Geometry check sheet. Reference: the model listing, model coordinates, mm. A direction names the side the tool comes from. Round coordinates to 2 decimals unless told otherwise and drop trailing zeros. Order: outer loops, then holes, each group sorted by start corner. A loop starts at its lowest first (then second) coordinate and runs counter-clockwise, first axis right, second up. Notation, with made-up numbers: (84.25, 87) - (100.25, 87) arc R25 cw to (100.25, 112) - close; hole circle Ø11 at (74.5, -31.75). An arc over 180 degrees is marked (long way). Return JSON: item names as keys, results as strings. Group by question number.
Q1. Sectioned sample at A-A, the plane y = -41. Record the cut outline in (x, z) (3 decimals).
Q2. Material ranges on line 1 along Y through (x, z) = (41, 2.75) (3 decimals); line 2 along Y through (x, z) = (-21, 9); line 3 along Y through (x, z) = (-23.5, 3), recorded low to high.
Q3. Gauge pin test, flat ends, axial feed: pin 1 Ø2 at (x, z) = (53, 1.5) entering from -Y; pin 2 Ø4 at (x, z) = (20.5, 5) entering from +Y; pin 3 Ø1 at (y, z) = (19, 5.5) entering from -X. Record the tip position at first contact, or that the pin passes through.
Q4. Sectioned sample at C-C, the plane x = -41. Record the cut outline in (y, z) (3 decimals), then the cut area to 3 significant figures.
Q5. Draft check along X on faces 1 (the flat face through (-45, 1, 5)), 2 (the flat face through (1, 45, 6)), 3 (the flat face through (-21.75, -20, 5)). Enter one of: pulls with the +X half, pulls with the -X half, needs draft (parallel to the pull), parting line crosses it, or undercut.
Q6. Tool access check on faces 4 (the flat face through (20, -18.25, 5)), 5 (the flat face through (45, -1, 5)), 6 (the flat face through (-1, 30, 0)). Record the directions out of +Z, -Z, +X, -X, +Y, -Y that give a thin tool (end or side, any length) a straight path to the whole face; none if there is none.
Q7. Sectioned sample at B-B, the plane z = 5. Give the number of separate pieces and of enclosed holes in the cut face, then the cut area to 3 significant figures.
Q8. Sectioned sample at D-D, the plane x = 12.5. Record the cut outline in (y, z), then the cut area to 4 significant figures.
```python
from build123d import *

# Parameters (mm, degrees)
F0_R     = 1.725
F0_W     = 3.5
F0_H     = 3.5
F1_DEPTH = 10
F3_DEPTH = 2


with BuildPart() as f1:
    # F0 (on Top) → F1 (new body)
    with BuildSketch(Plane.XY):
        Polygon((45, -45), (45, 0), (45, 45), (0, 45), (-45, 45), (-45, 0), (-45, -45), (0, -45), align=None)
        with Locations((-41, -41)):
            Circle(F0_R, mode=Mode.SUBTRACT)
        with Locations((-20, -20)):
            Rectangle(F0_W, F0_H, mode=Mode.SUBTRACT)
        with Locations((41, -41)):
            Circle(F0_R, mode=Mode.SUBTRACT)
        with Locations((20, -20)):
            Rectangle(F0_W, F0_H, mode=Mode.SUBTRACT)
        with Locations((-20, 20)):
            Rectangle(F0_W, F0_H, mode=Mode.SUBTRACT)
        with Locations((-41, 41)):
            Circle(F0_R, mode=Mode.SUBTRACT)
        with Locations((20, 20)):
            Rectangle(F0_W, F0_H, mode=Mode.SUBTRACT)
        with Locations((41, 41)):
            Circle(F0_R, mode=Mode.SUBTRACT)
    extrude(amount=F1_DEPTH)

    # F2 (on Top) → F3 (join)
    with BuildSketch(Plane.XY):
        Polygon((45, 102.5), (-45, 102.5), (-56.25, 102.5), (-56.25, 45), (56.25, 45), (56.25, 102.5), align=None)
    extrude(amount=F3_DEPTH)


solid = f1.part
```
Reply:
{
 "1": {"outline": "(-45, 0) - (-42.725, 0) - (-42.725, 10) - (-45, 10) - close; (-39.275, 0) - (39.275, 0) - (39.275, 10) - (-39.275, 10) - close; (42.725, 0) - (45, 0) - (45, 10) - (42.725, 10) - close"},
 "2": {"line 1": "-45 to -42.725, -39.275 to 39.275, 42.725 to 45", "line 2": "-45 to -21.75, -18.25 to 18.25, 21.75 to 45", "line 3": "-45 to 45"},
 "3": {"pin 1": "y = 45", "pin 2": "y = 45", "pin 3": "x = -45"},
 "4": {"outline": "(-45, 0) - (-42.725, 0) - (-42.725, 10) - (-45, 10) - close; (-39.275, 0) - (39.275, 0) - (39.275, 10) - (-39.275, 10) - close; (42.725, 0) - (102.5, 0) - (102.5, 2) - (45, 2) - (45, 10) - (42.725, 10) - close", "area": "946 mm^2"},
 "5": {"face 1": "pulls with the -X half", "face 2": "needs draft", "face 3": "undercut"},
 "6": {"face 4": "+Z, -Z", "face 5": "+Z, -Z, +X, -Y", "face 6": "-Z, +X, -X, +Y, -Y"},
 "7": {"separate pieces": "1", "enclosed holes": "8", "area": "8,010 mm^2"},
 "8": {"outline": "(-45, 0) - (102.5, 0) - (102.5, 2) - (45, 2) - (45, 10) - (-45, 10) - close", "area": "1,015 mm^2"}
}
